```python
from build123d import *

# Parameters (mm, degrees)
F0_R     = 104.775
F1_DEPTH = 28.575
F2_R     = 63.5
F3_DEPTH = 1.5875
F4_R     = 58.7375
F5_DEPTH = 14.2875
F5_TAPER = 3
F6_R     = 45.339
F7_DEPTH = 44.4510001
F9_D     = 22.225


with BuildPart() as f1:
    # F0 (on Top) → F1 (new body)
    with BuildSketch(Plane.XY):
        Circle(F0_R)
    extrude(amount=-F1_DEPTH)

    # F2 (on face) → F3 (join)
    with BuildSketch(Plane.XY):
        Circle(F2_R)
    extrude(amount=F3_DEPTH)

    # F4 (on face) → F5 (join)
    with BuildSketch(Plane(origin=(0, 0, -28.575), x_dir=(1, 0, 0), z_dir=(0, 0, -1))):
        Circle(F4_R)
    extrude(amount=F5_DEPTH, taper=F5_TAPER)

    # F6 (on face) → F7 (cut, through all)
    with BuildSketch(Plane.XY.offset(1.5875)):
        Circle(F6_R)
    extrude(amount=-F7_DEPTH, mode=Mode.SUBTRACT)

    # F9 (through all)
    with Locations(Plane.XY):
        with Locations((84.1375, 0), (59.4941968021, 59.4941968021), (0, 84.1375), (-59.4941968021, 59.4941968021), (-84.1375, 0), (-59.4941968021, -59.4941968021), (0, -84.1375), (59.4941968021, -59.4941968021)):
            Hole(F9_D / 2)


solid = f1.part
```
Check sheet for the modelled part. Datum: model origin and axes. Units: mm. A direction names the side the tool comes from. Round coordinates to 2 decimals unless told otherwise and drop trailing zeros. Write each loop counter-clockwise with the first axis right and the second up, starting at its lowest first coordinate (ties: lowest second). Pieces come first, ordered by that corner, then holes. Notation, with made-up numbers: (20.5, 39) -> (44.5, 39) arc R18 cw to (44.5, 72) -> close; hole circle Ø11 at (84.25, -15.5). An arc over 180 degrees is marked (long way). One line per question, with ' | ' between items. Start each with the question number.
1. Scan lines: line 1 along X through (y, z) = (55.5, -21.5); line 2 along X through (y, z) = (-57, -11.5); line 3 along Z through (x, y) = (-76, 10) (3 decimals). Record each from-to range of solid material in increasing order. Write a range as from..to.
2. Depth check by flat-ended pin: pin 1 (1 mm diameter, centred on x = -28.5, z = -33, fed in from +Y); pin 2 (3 mm diameter, centred on x = 3, z = -10.5, fed in from +Y); pin 3 (12 mm diameter, centred on x = 38.5, z = -12.5, fed in from -Y); pin 4 (18 mm diameter, centred on x = 0, y = 84.14, fed in from -Z). Enter the tip coordinate at first touch or a pass-through.
3. Set-up check for faces 1 (the face through (45, -45, -28.575)), 2 (the face through (45.1, -45.1, 0)), 3 (the face through (-35, 30, -42.862)): record each of +Z, -Z, +X, -X, +Y, -Y from which the full face is reachable in a straight line by a thin tool's end or side.
4. Release check for a two-part mould opening along Y. For faces 4 (the face through (-15, 43, 1.588)), 5 (the face through (95.24, 0.49, -14.49)), 6 (the face through (-13.77, -61.99, 0.78)) record: +Y half, -Y half, draft (parallel to the pull), parting line (faces both ways), or undercut.
5. Sectioned sample at B-B, the plane y = -80. Record the cut outline in (x, z) (3 decimals), then the cut area to 3 significant figures.
6. Sectioned sample at A-A, the plane x = 0. Count the separate pieces of the cut face and the enclosed holes in it, then the cut area to 3 significant figures.
7. Sectioned sample at C-C, the plane x = -81.5. Record the cut outline in (y, z) (3 decimals), then the cut area to 3 significant figures.
Taken from the geometry:
1) line 1: x = -88.87..-69.86, -49.12..49.12, 69.86..88.87 | line 2: x = -87.91..-70.32, -48.67..48.67, 70.32..87.91 | line 3: z = -28.575..0
2) pin 1: stops at y = 51.37 | pin 2: stops at y = 104.76 | pin 3: stops at y = -99.61 | pin 4: passes through
3) face 1: -Z | face 2: +Z | face 3: -Z, +X, -X, +Y, -Y
4) face 4: draft | face 5: undercut | face 6: parting line
5) outline: (-67.659, -28.575) -> (-10.314, -28.575) -> (-10.314, 0) -> (-67.659, 0) -> close; (10.314, -28.575) -> (67.659, -28.575) -> (67.659, 0) -> (10.314, 0) -> close | area: 3,280 mm^2
6) separate pieces: 4 | enclosed holes: 0 | area: 2,560 mm^2
7) outline: (-65.845, -28.575) -> (-10.795, -28.575) -> (-10.795, 0) -> (-65.845, 0) -> close; (10.795, -28.575) -> (65.845, -28.575) -> (65.845, 0) -> (10.795, 0) -> close | area: 3,150 mm^2
